Input: part model. Units: mm. Frame: model coordinates. A direction names the side the tool comes from. Coordinates: 2 decimals unless noted, no trailing zeros. Write each loop counter-clockwise with the first axis right and the second up, starting at its lowest first coordinate (ties: lowest second). Pieces come first, ordered by that corner, then holes. Notation, with made-up numbers: M -19,43 L 0,43 A21 cw 0,61 Z; hole C 78.25,15 d1. An arc over 180 degrees is marked long. Use one line per item in the form item = value.
from build123d import *

# Parameters (mm, degrees)
F0_W          = 35
F0_H          = 57
F1_DEPTH      = 31.5
F4_DEPTH      = 57.001
F5_DEPTH      = 35.0010001
F7_DEPTH      = 35.0010001
F9_DEPTH      = 2
F9_DEPTH_BACK = 37
F11_DEPTH     = 37.001
F12_W         = 6
F12_H         = 2.5
F13_DEPTH     = 4
F14_DEPTH     = 1


with BuildPart() as f1:
    # F0 (on Top) → F1 (new body)
    with BuildSketch(Plane.XY):
        with Locations((0.0945744105, -24.8016776452)):
            Rectangle(F0_W, F0_H)
    extrude(amount=F1_DEPTH)

    # F3 (on face) → F4 (cut, through all)
    with BuildSketch(Plane.XZ.offset(53.3016776452)):
        with BuildLine():
            add(Edge.make_bspline(
                [(0.0945744105, 2), (14.3839935729, 2), (7.2392839917, 17), (0.0945744105, 32), (-7.0501351708, 17), (-14.194844752, 2), (0.0945744105, 2)],
                knots=[0, 0, 0, 2.0943951024, 2.0943951024, 4.1887902048, 4.1887902048, 6.2831853072, 6.2831853072, 6.2831853072], degree=2, weights=[1, 0.5, 1, 0.5, 1, 0.5, 1]))
        make_face()
    extrude(amount=-F4_DEPTH, mode=Mode.SUBTRACT)

    # F2 (on face) → F5 (cut, through all)
    with BuildSketch(Plane.YZ.offset(17.5945744105)):
        with BuildLine():
            ThreePointArc((-53.3016776452, 0), (-35.9248296563, 21.279893434), (-10.4231016291, 31.5))
            Line((-10.4231016291, 31.5), (-53.3016776452, 31.5))
            Line((-53.3016776452, 31.5), (-53.3016776452, 0))
        make_face()
    extrude(amount=-F5_DEPTH, mode=Mode.SUBTRACT)

    # F6 (on face) → F7 (cut, through all)
    with BuildSketch(Plane.YZ.offset(17.5945744105)):
        with BuildLine():
            Line((3.6983223548, 0), (3.6983223548, 29))
            ThreePointArc((3.6983223548, 29), (-28.0042777095, 22.8678173622), (-50.8016776452, 0))
            Line((-50.8016776452, 0), (3.6983223548, 0))
        make_face()
    extrude(amount=-F7_DEPTH, mode=Mode.SUBTRACT)

    # F8 (on face) → F9 (join, two sides)
    with BuildSketch(Plane.YZ.offset(17.5945744105)) as f9_sk:
        with BuildLine():
            ThreePointArc((-49.9582016017, 1.5371667936), (-51.6783665277, 1.4810577961), (-50.8016776452, 0))
            ThreePointArc((-50.8016776452, 0), (-50.3860655446, 0.7719448198), (-49.9582016017, 1.5371667936))
        make_face()
        with BuildLine():
            ThreePointArc((-49.9582016017, 1.5371667936), (-50.3860655446, 0.7719448198), (-50.8016776452, 0))
            ThreePointArc((-50.8016776452, 0), (-50.094570864, 0.2928932188), (-49.8016776452, 1))
            ThreePointArc((-49.8016776452, 1), (-49.8416057615, 1.2797534241), (-49.9582016017, 1.5371667936))
        make_face()
    extrude(amount=F9_DEPTH)
    extrude(f9_sk.sketch, amount=-F9_DEPTH_BACK)

    # F10 (on face) → F11 (cut, through all)
    with BuildSketch(Plane.YZ.offset(17.5945744105)):
        with BuildLine():
            Line((-53.3016776452, 0), (-52.3163572735, 0))
            ThreePointArc((-52.3163572735, 0), (-52.6137174082, 0.8962393447), (-52.4206060402, 1.8205639696))
            ThreePointArc((-52.4206060402, 1.8205639696), (-52.8695111773, 0.9143323688), (-53.3016776452, 0))
        make_face()
    extrude(amount=-F11_DEPTH, mode=Mode.SUBTRACT)

    # F12 (on face) → F13 (join)
    with BuildSketch(Plane(origin=(0, 3.6983223548, 0), x_dir=(-1, 0, 0), z_dir=(0, 1, 0))):
        with Locations((-10.5945744105, 30.25)):
            Rectangle(F12_W, F12_H)
        with Locations((10.4054255895, 30.25)):
            Rectangle(F12_W, F12_H)
    extrude(amount=F13_DEPTH)

    # F14 (cut): faces of the model
    f14_faces = [f1.faces().sort_by_distance(p)[0] for p in [
        (10.5945744105, 5.6983223548, 29),
        (-10.4054255895, 5.6983223548, 29),
    ]]
    extrude(f14_faces, amount=-F14_DEPTH, mode=Mode.SUBTRACT)


solid = f1.part
(1) Section query A-A on x = -11.5. Return the cut outline in (y, z) (3 decimals), plus the area to 3 significant figures.
Computed:
outline = M -52.421,1.821 A1.815 ccw -52.316,0 L -50.802,0 A1 ccw -49.958,1.537 A55 cw 3.698,29 L 3.698,30 L 7.698,30 L 7.698,31.5 L -10.423,31.5 A55 ccw Z
area = 185 mm^2
(2) Section query C-C on z = 25. Return the cut outline in (x, y).
Computed:
outline = M -17.41,-30.13 L 17.59,-30.13 L 17.59,-23.52 L -17.41,-23.52 Z
(3) Section query B-B on y = -25. Return the cut outline in (x, z), plus the area to 3 significant figures.
Computed:
outline = M -17.41,24.35 L 17.59,24.35 L 17.59,27.52 L -17.41,27.52 Z
area = 111 mm^2
(4) Set-up query: faces 1 (the cylindrical face through (0.34, -52.613, 0.883)), 2 (the flat face through (0, -1, 31.5)), 3 (the flat face through (7.595, 6, 31)), 4 (the flat face through (-10, 6, 30)), 5 (the flat face through (-13.405, 6, 31)). Return all of +Z, -Z, +X, -X, +Y, -Y with unobstructed straight access to the full face (end or side cutting, diameter ignored); none if empty.
Computed:
face_1 = +X, -X, -Y
face_2 = +Z, +X, -X, +Y, -Y
face_3 = +Z, -Z, +Y
face_4 = -Z, +X, -X, +Y
face_5 = +Z, -Z, -X, +Y
(5) First-contact query: pin 1 Ø2 at (x, z) = (5, 30.5) entering from +Y; pin 2 Ø2 at (x, y) = (-7, -35) entering from +Z; pin 3 Ø1.5 at (x, y) = (-8.5, -44) entering from -Z. Flat tips, straight axial feed; report the tip coordinate or a pass-through.
Computed:
pin_1 = 3.7
pin_2 = 22.63
pin_3 = 9.12
(6) Line query: probe 1 along Z at (x, y) = (-1, -8); probe 2 along Y at (x, z) = (-15.5, 11); probe 3 along Y at (x, z) = (-7, 22.5). Output: solid intervals per line, ascending.
Computed:
probe_1 = 29 to 31.5
probe_2 = -46.56 to -43.15
probe_3 = -34.2 to -28.68
(7) Pull-direction query (X, two-part tool) for faces 6 (the flat face through (-7.405, 6, 31)), 7 (the flat face through (-19.405, -51, 1)), 8 (the flat face through (11, 7.698, 31)), 9 (the flat face through (13.595, 6, 31)); classes: pulls with the +X half, pulls with the -X half, needs draft (parallel to the pull), parting line crosses it, or undercut.
Computed:
face_6 = undercut
face_7 = pulls with the -X half
face_8 = needs draft
face_9 = pulls with the +X half
